from build123d import *

# Parameters (mm, degrees)
CROQUIS1_W              = 57.5
CROQUIS1_H              = 40
SALIENTE_EXTRUIR1_DEPTH = 4
CROQUIS3_W              = 4
CROQUIS3_H              = 40
SALIENTE_EXTRUIR3_DEPTH = 40
CORTAR_EXTRUIR1_REACH   = 6
CROQUIS5_R              = 2.25
CORTAR_EXTRUIR2_REACH   = 6
CROQUIS7_R              = 16.25
CROQUIS8_R              = 1.585
CORTAR_EXTRUIR3_DEPTH   = 4


with BuildPart() as part:
    # Croquis1 → Saliente-Extruir1 (new body)
    with BuildSketch(Plane(origin=(0, 0, 0), x_dir=(1, 0, 0), z_dir=(0, 1, 0))):
        Rectangle(CROQUIS1_W, CROQUIS1_H)
    extrude(amount=SALIENTE_EXTRUIR1_DEPTH)

    # Croquis3 → Saliente-Extruir3 (add)
    with BuildSketch(Plane(origin=(0, 4, 0), x_dir=(1, 0, 0), z_dir=(0, 1, 0))):
        with Locations((26.75, 0)):
            Rectangle(CROQUIS3_W, CROQUIS3_H)
    extrude(amount=SALIENTE_EXTRUIR3_DEPTH)

    # Croquis5 → Cortar-Extruir1 (cut, up to next)
    with BuildSketch(Plane.ZY.offset(-24.75), mode=Mode.PRIVATE) as cortar_extruir1_sk1:
        with Locations((-16.04, 38.8)):
            Circle(CROQUIS5_R)
    cortar_extruir1_tool1 = extrude(cortar_extruir1_sk1.sketch, amount=-CORTAR_EXTRUIR1_REACH, mode=Mode.PRIVATE) & part.part
    add(cortar_extruir1_tool1.solids().sort_by_distance((24.75, 38.8, -16.04))[0], mode=Mode.SUBTRACT)
    # Croquis5 → Cortar-Extruir1 (cut, up to next)
    with BuildSketch(Plane.ZY.offset(-24.75), mode=Mode.PRIVATE) as cortar_extruir1_sk2:
        with Locations((16.04, 38.8)):
            Circle(CROQUIS5_R)
    cortar_extruir1_tool2 = extrude(cortar_extruir1_sk2.sketch, amount=-CORTAR_EXTRUIR1_REACH, mode=Mode.PRIVATE) & part.part
    add(cortar_extruir1_tool2.solids().sort_by_distance((24.75, 38.8, 16.04))[0], mode=Mode.SUBTRACT)
    # Croquis5 → Cortar-Extruir1 (cut, up to next)
    with BuildSketch(Plane.ZY.offset(-24.75), mode=Mode.PRIVATE) as cortar_extruir1_sk3:
        with Locations((16.04, 9.2)):
            Circle(CROQUIS5_R)
    cortar_extruir1_tool3 = extrude(cortar_extruir1_sk3.sketch, amount=-CORTAR_EXTRUIR1_REACH, mode=Mode.PRIVATE) & part.part
    add(cortar_extruir1_tool3.solids().sort_by_distance((24.75, 9.2, 16.04))[0], mode=Mode.SUBTRACT)
    # Croquis5 → Cortar-Extruir1 (cut, up to next)
    with BuildSketch(Plane.ZY.offset(-24.75), mode=Mode.PRIVATE) as cortar_extruir1_sk4:
        with Locations((-16.04, 9.2)):
            Circle(CROQUIS5_R)
    cortar_extruir1_tool4 = extrude(cortar_extruir1_sk4.sketch, amount=-CORTAR_EXTRUIR1_REACH, mode=Mode.PRIVATE) & part.part
    add(cortar_extruir1_tool4.solids().sort_by_distance((24.75, 9.2, -16.04))[0], mode=Mode.SUBTRACT)

    # Croquis7 → Cortar-Extruir2 (cut, up to next)
    with BuildSketch(Plane.ZY.offset(-24.75), mode=Mode.PRIVATE) as cortar_extruir2_sk1:
        with Locations((0, 24)):
            Circle(CROQUIS7_R)
    cortar_extruir2_tool1 = extrude(cortar_extruir2_sk1.sketch, amount=-CORTAR_EXTRUIR2_REACH, mode=Mode.PRIVATE) & part.part
    add(cortar_extruir2_tool1.solids().sort_by_distance((24.75, 24, 0))[0], mode=Mode.SUBTRACT)

    # Croquis8 → Cortar-Extruir3 (cut)
    with BuildSketch(Plane.XZ):
        with Locations((-13.75, 15)):
            Circle(CROQUIS8_R)
        with Locations((13.75, 15)):
            Circle(CROQUIS8_R)
    cortar_extruir3 = extrude(amount=-CORTAR_EXTRUIR3_DEPTH, mode=Mode.SUBTRACT)

    # Simetr_a1: Cortar-Extruir3 across plane
    add(cortar_extruir3.mirror(Plane.XY), mode=Mode.SUBTRACT)


solid = part.part
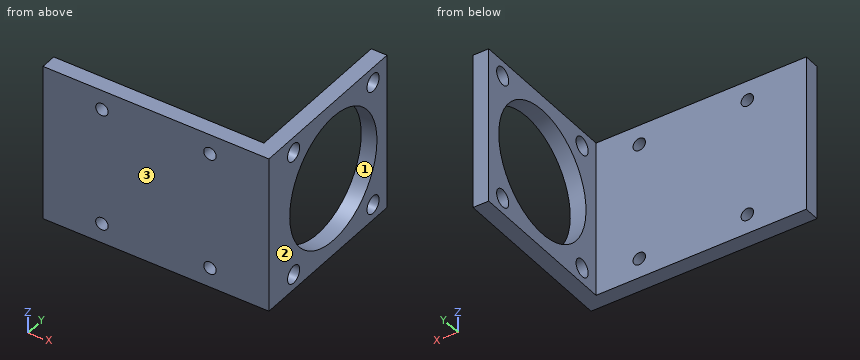
For this review, take the finished solid that the model builds, in its own axes (mm). Face numbers are marked on the shaded views. Coordinates: 2 decimals unless noted, no trailing zeros. Loops run counter-clockwise (first coordinate to the right, second up) from the corner with the lowest first, then second, coordinate; pieces in that order, holes last. Notation, with made-up numbers: (6, -16) - (13, -16) arc R19 cw to (13, -9) - close; hole circle Ø10 at (2.25, 29). An arc over 180 degrees is marked (long way). Use a Markdown table: item, result. Add a question column.
Item 1: For line 1 (Z direction, x = -13.75, y = 1) (3 decimals); line 2 (X direction, y = 2.4, z = -15) (3 decimals); line 3 (Y direction, x = -13.5, z = 4), list the stretches that pass through material, from the lowest coordinate up.
Item 2: We need section A-A (x = 13.75). Give the boundary of the cut face in (y, z) (3 decimals).
Item 3: We need section B-B (y = 24). Give the boundary of the cut face in (x, z).
Item 4: We need section D-D (y = 38.8). Give the boundary of the cut face in (x, z).
Item 5: Insertion check: pin 1 Ø4 at (y, z) = (38.8, -16.04) entering from +X; pin 2 Ø8 at (y, z) = (14, -8.5) entering from -X; pin 3 Ø5 at (x, z) = (-13.75, 15) entering from +Y. Each pin has a flat end and moves straight along its axis. Give the tip position at first contact, or say it passes through.
Item 6: Mouldability with a two-part tool opening along Y and no side actions: class the marked faces 1, 2 and 3 as pulls with the +Y half, pulls with the -Y half, needs draft (parallel to the pull), parting line crosses it, or undercut.
Item 7: We need section C-C (z = 6). Give the boundary of the cut face in (x, y), and give its area (3 significant figures).
Results list:
| question | item | result |
|---|---|---|
| 1 | line 1 | z = -20 to -16.585, -13.415 to 13.415, 16.585 to 20 |
| 1 | line 2 | x = -28.75 to -15.335, -12.165 to 12.165, 15.335 to 28.75 |
| 1 | line 3 | y = 0 to 4 |
| 2 | outline | (0, -20) - (4, -20) - (4, -16.585) - (0, -16.585) - close; (0, -13.415) - (4, -13.415) - (4, 13.415) - (0, 13.415) - close; (0, 16.585) - (4, 16.585) - (4, 20) - (0, 20) - close |
| 3 | outline | (24.75, -20) - (28.75, -20) - (28.75, -16.25) - (24.75, -16.25) - close; (24.75, 16.25) - (28.75, 16.25) - (28.75, 20) - (24.75, 20) - close |
| 4 | outline | (24.75, -20) - (28.75, -20) - (28.75, -18.29) - (24.75, -18.29) - close; (24.75, -13.79) - (28.75, -13.79) - (28.75, -6.71) - (24.75, -6.71) - close; (24.75, 6.71) - (28.75, 6.71) - (28.75, 13.79) - (24.75, 13.79) - close; (24.75, 18.29) - (28.75, 18.29) - (28.75, 20) - (24.75, 20) - close |
| 5 | pin 1 | passes through |
| 5 | pin 2 | stops at x = 24.75 |
| 5 | pin 3 | stops at y = 4 |
| 6 | face 1 | undercut |
| 6 | face 2 | needs draft |
| 6 | face 3 | pulls with the -Y half |
| 7 | outline | (-28.75, 0) - (28.75, 0) - (28.75, 8.9) - (24.75, 8.9) - (24.75, 4) - (-28.75, 4) - close; (24.75, 39.1) - (28.75, 39.1) - (28.75, 44) - (24.75, 44) - close |
| 7 | area | 269 mm^2 |
